from build123d import *

# Parameters (mm, degrees)
SKETCH_W          = 10
SKETCH_H          = 29.8
PAD_DEPTH         = 10
COPYSKETCH001_R   = 2
COPYSKETCH001_R_2 = 15
POCKET_DEPTH      = 10.001
FILLET_R          = 15


with BuildPart() as part:
    # Sketch → Pad (new body)
    with BuildSketch(Plane.XZ):
        Polygon((0, 0), (0, 57.4), (10, 57.4), (10, 87.2), (0, 87.2), (0, 117.2), (10, 117.2), (10, 147), (0, 147), (0, 177), (10, 177), (10, 200), (170, 200), (170, 177), (180, 177), (180, 200), (410, 200), (410, 177), (420, 177), (420, 147), (410, 147), (410, 117.2), (420, 117.2), (420, 87.2), (410, 87.2), (410, 57.4), (420, 57.4), (420, 0), align=None)
        with Locations((175, 132.1)):
            Rectangle(SKETCH_W, SKETCH_H, mode=Mode.SUBTRACT)
        with Locations((175, 72.3)):
            Rectangle(SKETCH_W, SKETCH_H, mode=Mode.SUBTRACT)
    extrude(amount=PAD_DEPTH)

    # CopySketch001 → Pocket (cut, through all)
    with BuildSketch(Plane.XZ):
        with Locations((73, 163.6)):
            Circle(COPYSKETCH001_R)
        with Locations((107, 163.6)):
            Circle(COPYSKETCH001_R)
        with Locations((107, 136.4)):
            Circle(COPYSKETCH001_R)
        with Locations((73, 136.4)):
            Circle(COPYSKETCH001_R)
        with Locations((90, 150)):
            Circle(COPYSKETCH001_R_2)
    extrude(amount=POCKET_DEPTH, mode=Mode.SUBTRACT)

    # Fillet
    fillet_edges = [part.edges().sort_by_distance(p)[0] for p in [
        (0, -5, 0),
    ]]
    fillet(fillet_edges, radius=FILLET_R)


solid = part.part
CAD build for the part. Positions are in the model's coordinates, mm. A direction names the side the tool comes from. Coordinates: 2 decimals unless noted, no trailing zeros. Order: outer loops, then holes, each group sorted by start corner. A loop starts at its lowest first (then second) coordinate and runs counter-clockwise, first axis right, second up.
Item 1: Band-saw the part on B-B on y = -4.75. Give the number of separate pieces and of enclosed holes in the cut face, plus the area to 3 significant figures.
Check sheet entries:
separate pieces: 1
enclosed holes: 7
area: 80,700 mm2
Item 2: 3-axis set-ups, long thin cutter, end or side, ignore diameter. For faces 4 (the face through (410, -5, 189)), 5 (the face through (175, -5, 57.4)), 6 (the face through (10, -5, 132)): which of +Z, -Z, +X, -X, +Y, -Y reach the whole face in a straight line?
Check sheet entries:
face 4: +Z, +X, +Y, -Y
face 5: +Y, -Y
face 6: -X, +Y, -Y
Item 3: Two-plate mould, pull along Z, no slides. Class faces 1 (the face through (293, -5, 200)), 2 (the face through (420, -5, 162)), 3 (the face through (410, -5, 73)): +Z half, -Z half, draft (parallel to the pull), parting line (faces both ways), or undercut.
Check sheet entries:
face 1: +Z half
face 2: draft
face 3: undercut
Item 4: Pin check, flat tips, straight feed: pin 1 Ø3 at (y, z) = (-3, 70.5) entering from +X; pin 2 Ø3 at (x, y) = (413.5, -6) entering from +Z; pin 3 Ø5 at (y, z) = (-4, 133) entering from -X. Stop position of each tip, or through.
Check sheet entries:
pin 1: stops at x = 410
pin 2: stops at z = 177
pin 3: stops at x = 10
Item 5: Band-saw the part on A-A on x = 90. List the corners of the cut face in (y, z).
Check sheet entries:
outline: (-10, 0) - (0, 0) - (0, 135) - (-10, 135) - close; (-10, 165) - (0, 165) - (0, 200) - (-10, 200) - close
Item 6: Drill centre lines: L1, parallel to Z at x = 107, y = -4; L2, parallel to X at y = -2.5, z = 136.4; L3, parallel to X at y = -6.5, z = 124. Where is each one in solid material? Low to high.
Check sheet entries:
L1: z = 0 to 134.4, 138.4 to 161.6, 165.6 to 200
L2: x = 10 to 71, 75 to 83.67, 96.33 to 105, 109 to 170, 180 to 410
L3: x = 10 to 170, 180 to 410
